Model file for the job. Use its own axes, mm. Face numbers are marked on the shaded views. A direction names the side the tool comes from. Coordinates: 2 decimals unless noted, no trailing zeros. Order: outer loops, then holes, each group sorted by start corner. A loop starts at its lowest first (then second) coordinate and runs counter-clockwise, first axis right, second up. Notation, with made-up numbers: M -24.75,64 L 16.25,64 A19 ccw 16.25,101 Z; hole C 51.5,51 d7. An arc over 180 degrees is marked long. Return JSON: item names as keys, results as strings.
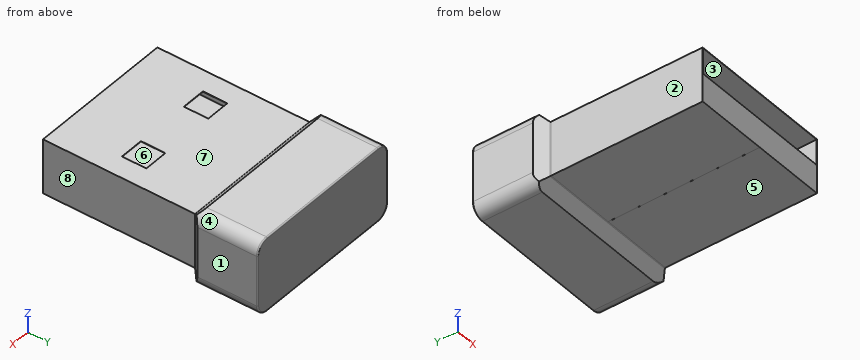
```python
from build123d import *

# Parameters (mm, degrees)
F0_W         = 12
F0_H         = 4.48
F1_DEPTH     = 5.75
F0_W_2       = 11.94
F0_H_2       = 2.3
F2_DEPTH     = 5.75
F3_W         = 13.63
F3_H         = 6.11
F3_W_2       = 12
F3_H_2       = 4.48
F3_W_3       = 11.94
F3_H_3       = 2.12
F4_DEPTH     = 6.73
F5_T4_DEPTH  = 22.7851914372
F5_T9_DEPTH  = 22.7851914372
F5_T14_DEPTH = 22.7851914372
F5_T19_DEPTH = 15.2651914372
F5_T24_DEPTH = 15.2651914372
F5_T29_DEPTH = 15.2651914372
F5_T34_DEPTH = 22.7851914372
F5_T39_DEPTH = 22.7851914372
F5_T44_DEPTH = 22.7851914372
F5_T49_DEPTH = 15.2651914372
F5_T54_DEPTH = 15.2651914372
F5_T59_DEPTH = 15.2651914372
F6_R         = 0.1
F7_R         = 1
F8_R         = 0.1
F9_W         = 2
F9_H         = 2
F10_DEPTH    = 2.15
F11_W        = 0.001
F11_H        = 12.4235786438
F12_DEPTH    = 0.3


# Not quite as in the source:
# - a fillet or chamfer that OpenCascade refuses, or shapes differently, is made with other operations: its cross-section is extruded or revolved along the edge and cut away or added


with BuildPart() as f1:
    # F0 (on Front) → F1 (new body, symmetric)
    with BuildSketch(Plane.XZ):
        Rectangle(F0_W, F0_H)
        Polygon((5.97, -2.21), (-5.97, -2.21), (-5.97, 0.09), (-5.97, 2.21), (5.97, 2.21), (5.97, 0.09), align=None, mode=Mode.SUBTRACT)
    extrude(amount=F1_DEPTH, both=True)

    # F0 (on Front) → F2 (join, symmetric)
    with BuildSketch(Plane.XZ):
        with Locations((0, -1.06)):
            Rectangle(F0_W_2, F0_H_2)
    extrude(amount=F2_DEPTH, both=True)

    # F3 (on face) → F4 (join)
    with BuildSketch(Plane(origin=(0, 5.75, 0), x_dir=(-1, 0, 0), z_dir=(0, 1, 0))):
        Rectangle(F3_W, F3_H)
        Rectangle(F3_W_2, F3_H_2, mode=Mode.SUBTRACT)
        Rectangle(F3_W_2, F3_H_2)
        with Locations((0, 1.15)):
            Rectangle(F3_W_3, F3_H_3, mode=Mode.SUBTRACT)
        with Locations((0, 1.15)):
            Rectangle(F3_W_3, F3_H_3)
    extrude(amount=F4_DEPTH)

    # F5: chamfer of 1.78 on 4 edges, made by hand


with BuildPart() as f5_tool2:
    # F5_s3 → F5_t4 (new body)
    with BuildSketch(Plane.YZ.offset(-11.3925957186)):
        Polygon((5.75, 1.275), (7.53, 3.055), (5.75, 3.055), align=None)
    extrude(amount=F5_T4_DEPTH)

    split(bisect_by=Plane.YZ.offset(-6), keep=Keep.BOTTOM)


with BuildPart() as f1_1:
    add(f1.part)

    # F5_t1: cut F5_tool2
    add(f5_tool2.part, mode=Mode.SUBTRACT)


with BuildPart() as f5_tool7:
    # F5_s8 → F5_t9 (new body)
    with BuildSketch(Plane.YZ.offset(-11.3925957186)):
        Polygon((5.75, 1.275), (7.53, 3.055), (5.75, 3.055), align=None)
    extrude(amount=F5_T9_DEPTH)

    split(bisect_by=Plane.XY.offset(2.24), keep=Keep.TOP)


with BuildPart() as f1_2:
    add(f1_1.part)

    # F5_t6: cut F5_tool7
    add(f5_tool7.part, mode=Mode.SUBTRACT)


with BuildPart() as f5_tool12:
    # F5_s13 → F5_t14 (new body)
    with BuildSketch(Plane.YZ.offset(-11.3925957186)):
        Polygon((5.75, 1.275), (7.53, 3.055), (5.75, 3.055), align=None)
    extrude(amount=F5_T14_DEPTH)

    split(bisect_by=Plane.YZ.offset(6), keep=Keep.TOP)


with BuildPart() as f1_3:
    add(f1_2.part)

    # F5_t11: cut F5_tool12
    add(f5_tool12.part, mode=Mode.SUBTRACT)


with BuildPart() as f5_tool17:
    # F5_s18 → F5_t19 (new body)
    with BuildSketch(Plane.XY.offset(7.6325957186)):
        Polygon((6.815, 7.53), (5.035, 5.75), (6.815, 5.75), align=None)
    extrude(amount=-F5_T19_DEPTH)

    split(bisect_by=Plane.YZ.offset(6), keep=Keep.TOP)


with BuildPart() as f1_4:
    add(f1_3.part)

    # F5_t16: cut F5_tool17
    add(f5_tool17.part, mode=Mode.SUBTRACT)


with BuildPart() as f5_tool22:
    # F5_s23 → F5_t24 (new body)
    with BuildSketch(Plane.XY.offset(7.6325957186)):
        Polygon((6.815, 7.53), (5.035, 5.75), (6.815, 5.75), align=None)
    extrude(amount=-F5_T24_DEPTH)

    split(bisect_by=Plane.XY.offset(2.24), keep=Keep.TOP)


with BuildPart() as f1_5:
    add(f1_4.part)

    # F5_t21: cut F5_tool22
    add(f5_tool22.part, mode=Mode.SUBTRACT)


with BuildPart() as f5_tool27:
    # F5_s28 → F5_t29 (new body)
    with BuildSketch(Plane.XY.offset(7.6325957186)):
        Polygon((6.815, 7.53), (5.035, 5.75), (6.815, 5.75), align=None)
    extrude(amount=-F5_T29_DEPTH)

    split(bisect_by=Plane.XY.offset(-2.24), keep=Keep.BOTTOM)


with BuildPart() as f1_6:
    add(f1_5.part)

    # F5_t26: cut F5_tool27
    add(f5_tool27.part, mode=Mode.SUBTRACT)


with BuildPart() as f5_tool32:
    # F5_s33 → F5_t34 (new body)
    with BuildSketch(Plane.YZ.offset(11.3925957186)):
        Polygon((7.53, -3.055), (5.75, -1.275), (5.75, -3.055), align=None)
    extrude(amount=-F5_T34_DEPTH)

    split(bisect_by=Plane.XY.offset(-2.24), keep=Keep.BOTTOM)


with BuildPart() as f1_7:
    add(f1_6.part)

    # F5_t31: cut F5_tool32
    add(f5_tool32.part, mode=Mode.SUBTRACT)


with BuildPart() as f5_tool37:
    # F5_s38 → F5_t39 (new body)
    with BuildSketch(Plane.YZ.offset(11.3925957186)):
        Polygon((7.53, -3.055), (5.75, -1.275), (5.75, -3.055), align=None)
    extrude(amount=-F5_T39_DEPTH)

    split(bisect_by=Plane.YZ.offset(6), keep=Keep.TOP)


with BuildPart() as f1_8:
    add(f1_7.part)

    # F5_t36: cut F5_tool37
    add(f5_tool37.part, mode=Mode.SUBTRACT)


with BuildPart() as f5_tool42:
    # F5_s43 → F5_t44 (new body)
    with BuildSketch(Plane.YZ.offset(11.3925957186)):
        Polygon((7.53, -3.055), (5.75, -1.275), (5.75, -3.055), align=None)
    extrude(amount=-F5_T44_DEPTH)

    split(bisect_by=Plane.YZ.offset(-6), keep=Keep.BOTTOM)


with BuildPart() as f1_9:
    add(f1_8.part)

    # F5_t41: cut F5_tool42
    add(f5_tool42.part, mode=Mode.SUBTRACT)


with BuildPart() as f5_tool47:
    # F5_s48 → F5_t49 (new body)
    with BuildSketch(Plane.XY.offset(-7.6325957186)):
        Polygon((-6.815, 7.53), (-5.035, 5.75), (-6.815, 5.75), align=None)
    extrude(amount=F5_T49_DEPTH)

    split(bisect_by=Plane.YZ.offset(-6), keep=Keep.BOTTOM)


with BuildPart() as f1_10:
    add(f1_9.part)

    # F5_t46: cut F5_tool47
    add(f5_tool47.part, mode=Mode.SUBTRACT)


with BuildPart() as f5_tool52:
    # F5_s53 → F5_t54 (new body)
    with BuildSketch(Plane.XY.offset(-7.6325957186)):
        Polygon((-6.815, 7.53), (-5.035, 5.75), (-6.815, 5.75), align=None)
    extrude(amount=F5_T54_DEPTH)

    split(bisect_by=Plane.XY.offset(-2.24), keep=Keep.BOTTOM)


with BuildPart() as f1_11:
    add(f1_10.part)

    # F5_t51: cut F5_tool52
    add(f5_tool52.part, mode=Mode.SUBTRACT)


with BuildPart() as f5_tool57:
    # F5_s58 → F5_t59 (new body)
    with BuildSketch(Plane.XY.offset(-7.6325957186)):
        Polygon((-6.815, 7.53), (-5.035, 5.75), (-6.815, 5.75), align=None)
    extrude(amount=F5_T59_DEPTH)

    split(bisect_by=Plane.XY.offset(2.24), keep=Keep.TOP)


with BuildPart() as f1_12:
    add(f1_11.part)

    # F5_t56: cut F5_tool57
    add(f5_tool57.part, mode=Mode.SUBTRACT)

    # F6
    f6_edges = [f1_12.edges().sort_by_distance(p)[0] for p in [
        (0, 6.715, 2.24),
        (6, 6.715, 0),
        (-6, 6.715, 0),
        (0, 6.715, -2.24),
    ]]
    fillet(f6_edges, radius=F6_R)

    # F7
    f7_edges = [f1_12.edges().sort_by_distance(p)[0] for p in [
        (-6.815, 10.005, -3.055),
        (-6.815, 10.005, 3.055),
        (6.815, 10.005, -3.055),
        (6.815, 10.005, 3.055),
    ]]
    fillet(f7_edges, radius=F7_R)

    # F8
    f8_edges = [f1_12.edges().sort_by_distance(p)[0] for p in [
        (0, 12.48, 3.055),
        (-6.522107, 12.48, 2.762107),
        (6.522107, 12.48, 2.762107),
        (-6.522107, 12.48, -2.762107),
        (-6.815, 12.48, 0),
        (0, 12.48, -3.055),
        (6.522107, 12.48, -2.762107),
        (6.815, 12.48, 0),
    ]]
    fillet(f8_edges, radius=F8_R)

    # F9 (on face) → F10 (cut, through all)
    with BuildSketch(Plane.XY.offset(2.24)):
        with Locations((-3.25, 0.35)):
            Rectangle(F9_W, F9_H)
        with Locations((3.25, 0.35)):
            Rectangle(F9_W, F9_H)
    extrude(amount=-F10_DEPTH, mode=Mode.SUBTRACT)

    # F11 (on face) → F12 (cut)
    with BuildSketch(Plane(origin=(0, 0, -2.24), x_dir=(1, 0, 0), z_dir=(0, 0, -1))):
        with Locations((0.0005, -0.4617893219)):
            Rectangle(F11_W, F11_H)
        with Locations((-0.0005, -0.4617893219)):
            Rectangle(F11_W, F11_H)
    extrude(amount=-F12_DEPTH, mode=Mode.SUBTRACT)


solid = f1_12.part
```
Item 1: Saw through at D-D (z = -1.25). Write the cut outline in (x, y) (3 decimals), and give its area (3 significant figures).
Check result:
{"outline": "M -6.815,7.53 L -6.029,6.744 A0.1 cw -6,6.674 L -6,-5.75 L 6,-5.75 L 6,6.674 A0.1 cw 6.029,6.744 L 6.815,7.53 L 6.815,12.38 A0.1 ccw 6.715,12.48 L -6.715,12.48 A0.1 ccw -6.815,12.38 Z", "area": "227 mm2"}
Item 2: Saw through at B-B (x = 2.75). Write the cut outline in (y, z) (3 decimals).
Check result:
{"outline": "M -5.75,-2.24 L 6.674,-2.24 A0.1 cw 6.744,-2.269 L 7.53,-3.055 L 12.38,-3.055 A0.1 ccw 12.48,-2.955 L 12.48,2.955 A0.1 ccw 12.38,3.055 L 7.53,3.055 L 6.744,2.269 A0.1 cw 6.674,2.24 L 1.35,2.24 L 1.35,2.21 L 5.75,2.21 L 5.75,0.09 L -5.75,0.09 Z; M -5.75,2.21 L -0.65,2.21 L -0.65,2.24 L -5.75,2.24 Z"}
Item 3: Drop flat-ended pins along their axis: pin 1 Ø8 at (x, y) = (-3.5, -1.5) entering from +Z; pin 2 Ø1.1 at (y, z) = (-2, 0.5) entering from -X; pin 3 Ø5 at (x, y) = (3, 1) entering from -Z. Give the stop position or say it passes through.
Check result:
{"pin 1": "stops at z = 2.24", "pin 2": "stops at x = -6", "pin 3": "stops at z = -2.24"}
Item 4: 3-axis set-ups, long thin cutter, end or side, ignore diameter. For the marked faces 1, 2, 3, 4 and 5: which of +Z, -Z, +X, -X, +Y, -Y reach the whole face in a straight line?
Check result:
{"face 1": "+Z, -Z, +X, +Y, -Y", "face 2": "+Z, -Z, -X, -Y", "face 3": "-Y", "face 4": "+Z, +X, +Y, -Y", "face 5": "-Z, +X, -X, -Y"}
Item 5: Wall check: line 1 (X direction, y = 2, z = -1.75); line 2 (Y direction, x = 3, z = 1); line 3 (Z direction, x = 3.75, y = 0). Give the ranges that are in metal, low to high.
Check result:
{"line 1": "x = -6 to 6", "line 2": "y = 5.75 to 12.48", "line 3": "z = -2.24 to 0.09"}
Item 6: Pull direction X, two halves, no side cores. Call the marked faces 6, 7 and 8: +X half, -X half, draft (parallel to the pull), parting line (faces both ways), or undercut.
Check result:
{"face 6": "undercut", "face 7": "draft", "face 8": "+X half"}
